from build123d import *

# Parameters (mm, degrees)
EXTRUDE_1_OUTLINE_W = 53
EXTRUDE_1_OUTLINE_H = 20
EXTRUDE_1_DEPTH     = 8.2
SKETCH_2_W          = 18
SKETCH_2_H          = 20
EXTRUDE_2_DEPTH     = 1
SKETCH_3_R          = 2.75
CUT_EXTRUDE_1_DEPTH = 30.48711583
SKETCH_4_W          = 17.5
SKETCH_4_H          = 4
EXTRUDE_3_DEPTH     = 8
FILLET_1_R          = 0.5


# Read off the part's stored shape, not the designer's step: 보스-돌출1
with BuildPart() as part:
    # 보스-돌출1 outline → 보스-돌출1 (new body)
    with BuildSketch(Plane.XY):
        Rectangle(EXTRUDE_1_OUTLINE_W, EXTRUDE_1_OUTLINE_H)
    extrude(amount=EXTRUDE_1_DEPTH)

    # 스케치2 → 보스-돌출2 (add)
    with BuildSketch(Plane.XY.offset(8.2)):
        Rectangle(SKETCH_2_W, SKETCH_2_H)
    extrude(amount=EXTRUDE_2_DEPTH)

    # 스케치3 → 컷-돌출1 (cut, through all)
    with BuildSketch(Plane.XY.offset(8.2)):
        with Locations((20.5, 0)):
            Circle(SKETCH_3_R)
        with Locations(Location((-20.5, 0, 0), (0, 0, 180))):
            Circle(SKETCH_3_R)
    extrude(amount=-CUT_EXTRUDE_1_DEPTH, mode=Mode.SUBTRACT)

    # 스케치4 → 보스-돌출3 (add)
    with BuildSketch(Plane.XY.offset(8.2)):
        with Locations((17.75, -8)):
            Rectangle(SKETCH_4_W, SKETCH_4_H)
        with Locations((17.75, 8)):
            Rectangle(SKETCH_4_W, SKETCH_4_H)
        with Locations((-17.75, 8)):
            Rectangle(SKETCH_4_W, SKETCH_4_H)
        with Locations((-17.75, -8)):
            Rectangle(SKETCH_4_W, SKETCH_4_H)
    extrude(amount=EXTRUDE_3_DEPTH)

    # 필렛1
    fillet_1_edges = [part.edges().sort_by_distance(p)[0] for p in [
        (26.5, -8, 16.2),
        (26.5, 8, 16.2),
        (-26.5, 8, 16.2),
        (-26.5, -8, 16.2),
    ]]
    fillet(fillet_1_edges, radius=FILLET_1_R)


solid = part.part
Can you work these out from the model? Positions are in its coordinate system, mm. A direction names the side the tool comes from. Give positions to 0.01 mm unless a question says otherwise; leave off trailing zeros. Write each loop counter-clockwise with the first axis right and the second up, starting at its lowest first coordinate (ties: lowest second). Pieces come first, ordered by that corner, then holes. Notation, with made-up numbers: (-1.5, 68.5) -> (32.5, 68.5) arc R24 ccw to (32.5, 88.5) -> close; hole circle Ø9 at (-3, 75). An arc over 180 degrees is marked (long way). Answer as a JSON object with one key per item and string values. Group by question number.
Item 1: Suppose I cut it at C-C (x = -20.5). Please give me the cut outline in (y, z), plus the area to 3 significant figures.
Item 2: I'm going to push flat-ended pins straight in: P1, Ø0.5, axis at y = -1.5, z = 8.5, coming from the -X side; P2, Ø9.5, axis at x = -21, y = -1, coming from the +Z side; P3, Ø1.1, axis at y = 3, z = 9, coming from the +X side. Where does each tip first touch, or does it pass through?
Item 3: Suppose I cut it at A-A (y = 0). Please give me the cut outline in (x, z), plus the area to 3 significant figures.
Item 4: Please list where these lines run through material, in increasing order: line 1 (X direction, y = -6.75, z = 13.75); line 2 (Y direction, x = 9.5, z = 9.75); line 3 (Y direction, x = 20.5, z = 5). Write a range as [from, to].
Item 5: Suppose I cut it at D-D (x = 16). Please give me the cut outline in (y, z), plus the area to 3 significant figures.
Item 6: Suppose I cut it at B-B (z = 14). Please give me the cut outline in (x, y), plus the area to 3 significant figures.
Item 7: For faces 1 (the face through (9, 0, 9)), 2 (the face through (-9, 0, 9)), 3 (the face through (0, 0, 9.2)), which set-ups out of +Z, -Z, +X, -X, +Y, -Y let a thin tool reach every point of the face, with its end or its side?
Findings:
{
 "1": {"outline": "(-10, 0) -> (-2.75, 0) -> (-2.75, 8.2) -> (-6, 8.2) -> (-6, 16.2) -> (-10, 16.2) -> close; (2.75, 0) -> (10, 0) -> (10, 16.2) -> (6, 16.2) -> (6, 8.2) -> (2.75, 8.2) -> close", "area": "183 mm²"},
 "2": {"P1": "stops at x = -9", "P2": "stops at z = 8.2", "P3": "stops at x = 9"},
 "3": {"outline": "(-26.5, 0) -> (-23.25, 0) -> (-23.25, 8.2) -> (-26.5, 8.2) -> close; (-17.75, 0) -> (17.75, 0) -> (17.75, 8.2) -> (9, 8.2) -> (9, 9.2) -> (-9, 9.2) -> (-9, 8.2) -> (-17.75, 8.2) -> close; (23.25, 0) -> (26.5, 0) -> (26.5, 8.2) -> (23.25, 8.2) -> close", "area": "362 mm²"},
 "4": {"line 1": "x = [-26.5, -9], [9, 26.5]", "line 2": "y = [-10, -6], [6, 10]", "line 3": "y = [-10, -2.75], [2.75, 10]"},
 "5": {"outline": "(-10, 0) -> (10, 0) -> (10, 16.2) -> (6, 16.2) -> (6, 8.2) -> (-6, 8.2) -> (-6, 16.2) -> (-10, 16.2) -> close", "area": "228 mm²"},
 "6": {"outline": "(-26.5, -10) -> (-9, -10) -> (-9, -6) -> (-26.5, -6) -> close; (-26.5, 6) -> (-9, 6) -> (-9, 10) -> (-26.5, 10) -> close; (9, -10) -> (26.5, -10) -> (26.5, -6) -> (9, -6) -> close; (9, 6) -> (26.5, 6) -> (26.5, 10) -> (9, 10) -> close", "area": "280 mm²"},
 "7": {"face 1": "+Z, +X", "face 2": "+Z, -X", "face 3": "+Z, +Y, -Y"}
}
